Work out the finished part from the listing and answer in its coordinate system (mm). Coordinates: 2 decimals unless noted, no trailing zeros. Order: outer loops, then holes, each group sorted by start corner. A loop starts at its lowest first (then second) coordinate and runs counter-clockwise, first axis right, second up. Notation, with made-up numbers: (-15.75, -3) - (38.25, -3) arc R11 ccw to (38.25, 2) - close; hole circle Ø7 at (-0.75, 0). An arc over 180 degrees is marked (long way). Answer as a JSON object with one key per item and string values. Group by question number.
1) Section C-C (y = 19) is taken. Give the vertices of the cut face in (x, z).
2) This flat-tipped pin is pushed along its axis until it touches: P1, Ø1.5, axis at x = 539, z = -163.5, coming from the +Y side. Where does it stop, or does it pass through?
3) The mould has two halves that part along X. Classify faces 1 (the face through (600, 27, -148)), 2 (the face through (358.31, 27.88, -52.82)), 3 (the face through (0, 27, -148)), 4 (the face through (296, 27, 0)): released by +X, released by -X, zero draft, split by the parting line, or undercut.
4) Section B-B (x = 550) is taken. Give the vertices of the cut face in (y, z), plus the area to 3 significant figures.
5) Section D-D (x = 229) is taken. Give the vertices of the cut face in (y, z).
6) Section A-A (z = -150) is taken. Give the vertices of the cut face in (x, y), plus the area to 3 significant figures.
7) Find the intervals of material crossed by line 1 along X through (y, z) = (20, -250); line 2 along X through (y, z) = (36.5, -152); line 3 along Z through (x, y) = (239.5, 42.5), in increasing order.
from build123d import *

# Parameters (mm, degrees)
SKETCH_1_W          = 600
SKETCH_1_H          = 300
EXTRUDE_1_DEPTH     = 55
SKETCH_2_R          = 19.5
SKETCH_2_R_2        = 13
CUT_EXTRUDE_1_DEPTH = 674.071318658


with BuildPart() as part:
    # 草图1 → 凸台-拉伸1 (new body)
    with BuildSketch(Plane(origin=(0, 0, 0), x_dir=(1, 0, 0), z_dir=(0, 1, 0))):
        with Locations((300, 150)):
            Rectangle(SKETCH_1_W, SKETCH_1_H)
    extrude(amount=EXTRUDE_1_DEPTH)

    # 草图2 → 切除-拉伸1 (cut, through all)
    with BuildSketch(Plane(origin=(0, 55, 0), x_dir=(1, 0, 0), z_dir=(0, 1, 0))):
        with Locations(Location((50, 150, 0), (0, 0, 270))):
            Circle(SKETCH_2_R)
        with Locations(Location((550, 150, 0), (0, 0, 270))):
            Circle(SKETCH_2_R)
        with Locations(Location((371, 250, 0), (0, 0, 270))):
            Circle(SKETCH_2_R_2)
        with Locations(Location((229, 250, 0), (0, 0, 270))):
            Circle(SKETCH_2_R_2)
        with Locations(Location((371, 50, 0), (0, 0, 270))):
            Circle(SKETCH_2_R_2)
        with Locations(Location((229, 50, 0), (0, 0, 270))):
            Circle(SKETCH_2_R_2)
    extrude(amount=-CUT_EXTRUDE_1_DEPTH, mode=Mode.SUBTRACT)


solid = part.part
Report:
{
 "1": {"outline": "(0, -300) - (600, -300) - (600, 0) - (0, 0) - close; hole circle Ø39 at (50, -150); hole circle Ø26 at (229, -250); hole circle Ø26 at (229, -50); hole circle Ø26 at (371, -250); hole circle Ø26 at (371, -50); hole circle Ø39 at (550, -150)"},
 "2": {"P1": "passes through"},
 "3": {"face 1": "released by +X", "face 2": "undercut", "face 3": "released by -X", "face 4": "zero draft"},
 "4": {"outline": "(0, -300) - (55, -300) - (55, -169.5) - (0, -169.5) - close; (0, -130.5) - (55, -130.5) - (55, 0) - (0, 0) - close", "area": "14,400 mm²"},
 "5": {"outline": "(0, -300) - (55, -300) - (55, -263) - (0, -263) - close; (0, -237) - (55, -237) - (55, -63) - (0, -63) - close; (0, -37) - (55, -37) - (55, 0) - (0, 0) - close"},
 "6": {"outline": "(0, 0) - (30.5, 0) - (30.5, 55) - (0, 55) - close; (69.5, 0) - (530.5, 0) - (530.5, 55) - (69.5, 55) - close; (569.5, 0) - (600, 0) - (600, 55) - (569.5, 55) - close", "area": "28,700 mm²"},
 "7": {"line 1": "x = 0 to 216, 242 to 358, 384 to 600", "line 2": "x = 0 to 30.6, 69.4 to 530.6, 569.4 to 600", "line 3": "z = -300 to -257.66, -242.34 to -57.66, -42.34 to 0"}
}
